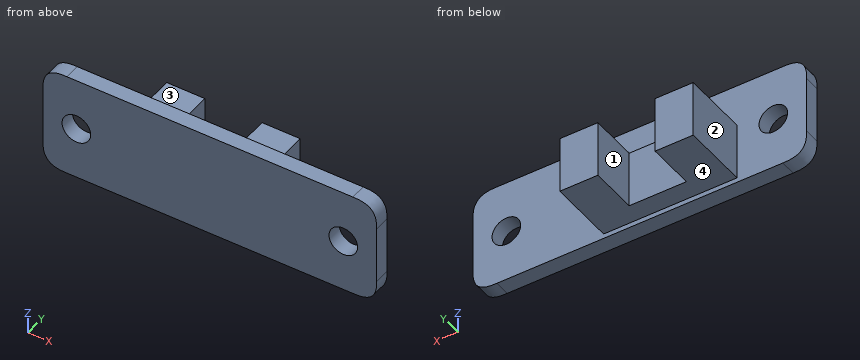
from build123d import *

# Parameters (mm, degrees)
SKETCH1_W           = 35
SKETCH1_H           = 11
SKETCH1_R           = 1.5
BOSS_EXTRUDE1_DEPTH = 1.65
FILLET1_SIZE        = 2.5
BOSS_EXTRUDE2_START = 1.65
SKETCH1_3_W         = 14
SKETCH1_3_H         = 6
BOSS_EXTRUDE2_DEPTH = 2
BOSS_EXTRUDE3_START = 3.65
SKETCH1_4_W         = 4
SKETCH1_4_H         = 5
SKETCH1_4_H_2       = 1
BOSS_EXTRUDE3_DEPTH = 5


with BuildPart() as part:
    # Sketch1 → Boss-Extrude1 (new body)
    with BuildSketch(Plane(origin=(0, 0, 0), x_dir=(1, 0, 0), z_dir=(0, 1, 0))):
        with Locations((17.5, 5.5)):
            Rectangle(SKETCH1_W, SKETCH1_H)
        with Locations(Location((3.5, 5.5, 0), (0, 0, 270))):
            Circle(SKETCH1_R, mode=Mode.SUBTRACT)
        with Locations(Location((31.5, 5.5, 0), (0, 0, 270))):
            Circle(SKETCH1_R, mode=Mode.SUBTRACT)
    extrude(amount=BOSS_EXTRUDE1_DEPTH)

    # Fillet1
    # a fillet whose section is not a circle: 2.5 mm, written as the material it takes off along each edge
    with BuildSketch(Plane(origin=(0, -6.25, -11), x_dir=(1, 0, 0), z_dir=(0, 1, 0)), Plane(origin=(35, -6.25, -11), x_dir=(0, 0, 1), z_dir=(0, 1, 0)), Plane(origin=(35, -6.25, 0), x_dir=(-1, 0, 0), z_dir=(0, 1, 0))) as fillet1_piece_1:
        with BuildLine():
            add(Edge.make_bspline([(FILLET1_SIZE, 0), (FILLET1_SIZE * 0.831801948466, 0), (FILLET1_SIZE * 0.663603896932, 0), (FILLET1_SIZE * 0.292893218813, -FILLET1_SIZE * 0.0716919198361), (FILLET1_SIZE * 0.0716919198361, -FILLET1_SIZE * 0.292893218813), (0, -FILLET1_SIZE * 0.663603896932), (0, -FILLET1_SIZE * 0.831801948466), (0, -FILLET1_SIZE)], knots=[0, 0, 0, 0, 0, 0, 0.5, 0.5, 1, 1, 1, 1, 1, 1], degree=5))
            Line((0, -FILLET1_SIZE), (0, 0))
            Line((0, 0), (FILLET1_SIZE, 0))
        make_face()
    extrude(amount=14.15, mode=Mode.SUBTRACT)
    with BuildSketch(Plane(origin=(0, -6.25, 0), x_dir=(1, 0, 0), z_dir=(0, 1, 0))) as fillet1_piece_2:
        with BuildLine():
            add(Edge.make_bspline([(FILLET1_SIZE, 0), (FILLET1_SIZE * 0.831801948466, 0), (FILLET1_SIZE * 0.663603896932, 0), (FILLET1_SIZE * 0.292893218813, FILLET1_SIZE * 0.0716919198361), (FILLET1_SIZE * 0.0716919198361, FILLET1_SIZE * 0.292893218813), (0, FILLET1_SIZE * 0.663603896932), (0, FILLET1_SIZE * 0.831801948466), (0, FILLET1_SIZE)], knots=[0, 0, 0, 0, 0, 0, 0.5, 0.5, 1, 1, 1, 1, 1, 1], degree=5))
            Line((0, FILLET1_SIZE), (0, 0))
            Line((0, 0), (FILLET1_SIZE, 0))
        make_face()
    extrude(amount=14.15, mode=Mode.SUBTRACT)

    # Sketch1<3> → Boss-Extrude2 (add)
    with BuildSketch(Plane(origin=(0, 0, 0), x_dir=(1, 0, 0), z_dir=(0, 1, 0)).offset(BOSS_EXTRUDE2_START)):
        with Locations((14.3, 7.5)):
            Rectangle(SKETCH1_3_W, SKETCH1_3_H)
    extrude(amount=BOSS_EXTRUDE2_DEPTH)

    # Sketch1<4> → Boss-Extrude3 (add)
    with BuildSketch(Plane(origin=(0, 0, 0), x_dir=(1, 0, 0), z_dir=(0, 1, 0)).offset(BOSS_EXTRUDE3_START)):
        with Locations((9.3, 8)):
            Rectangle(SKETCH1_4_W, SKETCH1_4_H)
        with Locations((19.3, 8)):
            Rectangle(SKETCH1_4_W, SKETCH1_4_H)
        with Locations((9.3, 5)):
            Rectangle(SKETCH1_4_W, SKETCH1_4_H_2)
        with Locations((19.3, 5)):
            Rectangle(SKETCH1_4_W, SKETCH1_4_H_2)
    extrude(amount=BOSS_EXTRUDE3_DEPTH)


solid = part.part
Can you work these out from the model? Positions are in its coordinate system, mm. Face numbers are marked on the shaded views. A direction names the side the tool comes from. Coordinates: 2 decimals unless noted, no trailing zeros. Write each loop counter-clockwise with the first axis right and the second up, starting at its lowest first coordinate (ties: lowest second). Pieces come first, ordered by that corner, then holes.
Q1. Imagine slicing it at A-A, the plane z = -5.5. List the corners of the cut face in (x, y) for me, plus the area to 3 significant figures.
Results found:
outline: (0, 0) - (2, 0) - (2, 1.65) - (0, 1.65) - close; (5, 0) - (30, 0) - (30, 1.65) - (21.3, 1.65) - (21.3, 8.65) - (17.3, 8.65) - (17.3, 3.65) - (11.3, 3.65) - (11.3, 8.65) - (7.3, 8.65) - (7.3, 1.65) - (5, 1.65) - close; (33, 0) - (35, 0) - (35, 1.65) - (33, 1.65) - close
area: 116 mm2
Q2. Imagine slicing it at C-C, the plane x = 20. List the corners of the cut face in (y, z) for me, plus the area to 4 significant figures.
Results found:
outline: (0, -11) - (1.65, -11) - (1.65, -10.5) - (8.65, -10.5) - (8.65, -4.5) - (1.65, -4.5) - (1.65, 0) - (0, 0) - close
area: 60.15 mm2
Q3. Which directions (+Z, -Z, +X, -X, +Y, -Y) give clear straight access to the entire face, cutting with the end or side of a thin tool? Please do the marked faces 1, 2, 3 and 4.
Results found:
face 1: +Z, -Z, +Y
face 2: +Z, -Z, -X, +Y
face 3: +Z, +X, -X, +Y
face 4: -Z, +X, -X, +Y
Q4. Please list where these lines run through material, in increasing order: L1, parallel to X at y = 1.15, z = -5.5; L2, parallel to X at y = 5, z = -9.5; L3, parallel to Y at x = 24, z = -3.5.
Results found:
L1: x = 0 to 2, 5 to 30, 33 to 35
L2: x = 7.3 to 11.3, 17.3 to 21.3
L3: y = 0 to 1.65
Q5. Imagine slicing it at D-D, the plane z = -8. List the corners of the cut face in (x, y) for me, plus the area to 3 significant figures.
Results found:
outline: (0, 0) - (35, 0) - (35, 1.65) - (21.3, 1.65) - (21.3, 8.65) - (17.3, 8.65) - (17.3, 3.65) - (11.3, 3.65) - (11.3, 8.65) - (7.3, 8.65) - (7.3, 1.65) - (0, 1.65) - close
area: 126 mm2
Q6. Imagine slicing it at B-B, the plane x = 3.5. List the corners of the cut face in (y, z) for me, plus the area to 3 significant figures.
Results found:
outline: (0, -11) - (1.65, -11) - (1.65, -7) - (0, -7) - close; (0, -4) - (1.65, -4) - (1.65, 0) - (0, 0) - close
area: 13.2 mm2
Q7. For P1, Ø5, axis at x = 16, y = 4.5, coming from the +Z side; P2, Ø3, axis at y = 5, z = -7, coming from the +X side; P3, Ø3, axis at y = 4, z = -6.5, coming from the -X side, each with a flat end and sliding along its axis, tell me the tip position at first contact or that it passes through.
Results found:
P1: stops at z = -4.5
P2: stops at x = 21.3
P3: stops at x = 7.3
